Geometry: see drawing. Coordinates: mm, zero at the bounding-box minimum. Round coordinates to 2 decimals unless told otherwise and drop trailing zeros. Loops run counter-clockwise (first coordinate to the right, second up) from the corner with the lowest first, then second, coordinate; pieces in that order, holes last. Notation, with made-up numbers: (17, 52) - (51, 52) arc R36 cw to (51, 87) - close; hole circle Ø3 at (-28.5, -27.75). An arc over 180 degrees is marked (long way). Write item = value, one per line. Start each with the question number.
Item 1: Line query: line 1 (Y direction, x = 86, z = 1.9); line 2 (X direction, y = 83.5, z = 3.2); line 3 (X direction, y = 70.5, z = 0.35). Output: solid intervals per line, ascending. Write a range as from..to.
Item 2: First-contact query: pin 1 (1.9 mm diameter, centred on x = 35.5, z = 2.5, fed in from -Y); pin 2 (2 mm diameter, centred on x = 151.5, z = 1, fed in from -Y). Flat tips, straight axial feed; report the tip coordinate or a pass-through.
Item 3: Section C-C (x = 83). Return loops of the section in (y, z).
Item 4: Section B-B (z = 2.25). Count the separate pieces of the cut face and the enclosed holes in it, plus the area to 3 significant figures.
Item 5: Section A-A (y = 95). Return loops of the section in (x, z).
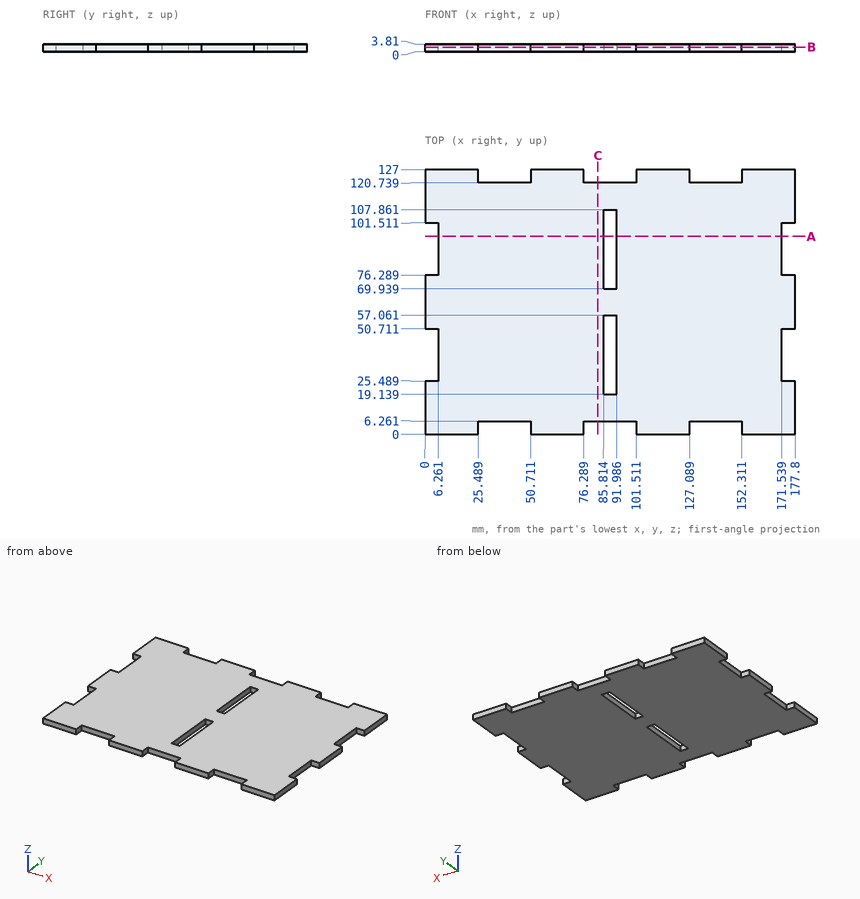
Taken from the geometry:
q1.line_1 = 6.26..19.14, 57.06..69.94, 107.86..120.74
q1.line_2 = 6.26..85.81, 91.99..171.54
q1.line_3 = 0..85.81, 91.99..177.8
q2.pin_1 = 6.26
q2.pin_2 = 0
q3.outline = (6.26, 0) - (120.74, 0) - (120.74, 3.81) - (6.26, 3.81) - close
q4.separate_pieces = 1
q4.enclosed_holes = 2
q4.area = 20,500 mm^2
q5.outline = (6.26, 0) - (85.81, 0) - (85.81, 3.81) - (6.26, 3.81) - close; (91.99, 0) - (171.54, 0) - (171.54, 3.81) - (91.99, 3.81) - close
